```python
from build123d import *

# Parameters (mm, degrees)
F0_W      = 438.5
F0_H      = 130
F1_DEPTH  = 14
F2_W      = 30
F2_H      = 10
F3_DEPTH  = 130
F4_W      = 11
F4_H      = 16
F5_DEPTH  = 130
F6_W      = 42.5
F6_H      = 23.3528089888
F6_H_2    = 62.2471910113
F7_DEPTH  = 25
F8_R      = 2.5
F9_DEPTH  = 25
F10_R     = 2.5
F11_DEPTH = 468.501
F12_SIZE  = 3.49999


# Not quite as in the source:
# - a fillet or chamfer is up to 0.001 mm smaller than in the source, because OpenCascade refuses the exact size
# - a feature names something its author has since deleted; it is built from what else it names


with BuildPart() as f1:
    # F0 (on Front) → F1 (new body)
    with BuildSketch(Plane.XZ):
        with Locations((219.25, 65)):
            Rectangle(F0_W, F0_H)
    extrude(amount=F1_DEPTH)

    # F2 (on face) → F3 (join, through all)
    with BuildSketch(Plane.XY.offset(130)):
        with Locations((453.5, -9)):
            Rectangle(F2_W, F2_H)
        with Locations((-15, -9)):
            Rectangle(F2_W, F2_H)
    extrude(amount=-F3_DEPTH)

    # F4 (on face) → F5 (join, through all)
    with BuildSketch(Plane.XY.offset(130)):
        with Locations((5.5, 8)):
            Rectangle(F4_W, F4_H)
        with Locations((433, 8)):
            Rectangle(F4_W, F4_H)
    extrude(amount=-F5_DEPTH)

    # F6 (on face) → F7 (cut)
    with BuildSketch(Plane.XZ.offset(14)):
        Polygon((24.75, 120), (24.75, 95), (14.75, 95), (14.75, 57.7528089887), (24.75, 57.7528089887), (67.25, 57.7528089887), (67.25, 120), align=None)
        with Locations((46, 21.6764044942)):
            Rectangle(F6_W, F6_H)
        with Locations((101.4, 41.1235955055)):
            Rectangle(F6_W, F6_H_2)
        with Locations((143.9, 41.1235955055)):
            Rectangle(F6_W, F6_H_2)
        with Locations((101.4, 108.3235955056)):
            Rectangle(F6_W, F6_H)
        with Locations((143.9, 108.3235955056)):
            Rectangle(F6_W, F6_H)
        with Locations((199.3, 88.8764044943)):
            Rectangle(F6_W, F6_H_2)
        with Locations((241.8, 88.8764044943)):
            Rectangle(F6_W, F6_H_2)
        with Locations((199.3, 21.6764044942)):
            Rectangle(F6_W, F6_H)
        with Locations((241.8, 21.6764044942)):
            Rectangle(F6_W, F6_H)
        with Locations((297.2, 41.1235955055)):
            Rectangle(F6_W, F6_H_2)
        with Locations((339.7, 41.1235955055)):
            Rectangle(F6_W, F6_H_2)
        with Locations((339.7, 108.3235955056)):
            Rectangle(F6_W, F6_H)
        with Locations((297.2, 108.3235955056)):
            Rectangle(F6_W, F6_H)
        Polygon((416.35, 120), (373.85, 120), (373.85, 57.7528089887), (427.35, 57.7528089887), (427.35, 95), (416.35, 95), align=None)
        with Locations((395.1, 21.6764044942)):
            Rectangle(F6_W, F6_H)
    extrude(amount=-F7_DEPTH, mode=Mode.SUBTRACT)

    # F8 (on face) → F9 (cut)
    with BuildSketch(Plane(origin=(0, -4, 0), x_dir=(-1, 0, 0), z_dir=(0, 1, 0))):
        with Locations((-448.5, 115)):
            Circle(F8_R)
        with Locations((-448.5, 15)):
            Circle(F8_R)
        with Locations((10, 115)):
            Circle(F8_R)
        with Locations((10, 15)):
            Circle(F8_R)
    extrude(amount=-F9_DEPTH, mode=Mode.SUBTRACT)

    # F10 (on face) → F11 (cut, through all)
    with BuildSketch(Plane.YZ.offset(438.5)):
        with Locations((6, 115)):
            Circle(F10_R)
        with Locations((6, 15)):
            Circle(F10_R)
        with Locations((6, 65)):
            Circle(F10_R)
    extrude(amount=-F11_DEPTH, mode=Mode.SUBTRACT)

    # F12 (size 3.5 in the source; OpenCascade refuses exactly that, so slightly less here)
    f12_edges = [f1.edges().sort_by_distance(p)[0] for p in [
        (451, -14, 115),
        (451, -14, 15),
        (-7.5, -14, 115),
        (-7.5, -14, 15),
        (427.5, 3.5, 115),
        (427.5, 3.5, 65),
        (427.5, 3.5, 15),
        (11, 3.5, 115),
        (11, 3.5, 65),
        (11, 3.5, 15),
    ]]
    chamfer(f12_edges, length=F12_SIZE)


solid = f1.part
```
Geometry: final body of the model. Coordinates: model frame, mm. A direction names the side the tool comes from. Give positions to 0.01 mm unless a question says otherwise; leave off trailing zeros. Write each loop counter-clockwise with the first axis right and the second up, starting at its lowest first coordinate (ties: lowest second). Pieces come first, ordered by that corner, then holes.
1. Reachability of faces 4 (the conical face through (430.83, 5.421, 62.394)), 5 (the flat face through (416.35, -7, 107)), 6 (the flat face through (271, -5, 0)) from +Z, -Z, +X, -X, +Y, -Y: full face, straight path, thin tool, end or side. Return the list, or none.
2. Line query: probe 1 along X at (y, z) = (-3.5, 93); probe 2 along Z at (x, y) = (205, -6.25); probe 3 along X at (y, z) = (-3.25, 43). Output: solid intervals per line, ascending.
3. Section query A-A, the plane z = 83.5. Return loops of the section in (x, y), then the cut area to 3 significant figures.
4. Draft query along X for faces 1 (the flat face through (5, 16, 66)), 2 (the flat face through (20, -7, 95)), 3 (the flat face through (178.05, -7, 88)). Return one class per face: released by +X, released by -X, zero draft, split by the parting line, or undercut.
5. Section query B-B, the plane x = 102. Return loops of the section in (y, z), then the cut area to 3 significant figures.
6. Pin query (flat end, axial travel): P1, Ø24, axis at x = 452, z = 41, coming from the +Y side; P2, Ø1.5, axis at y = 10, z = 84.5, coming from the +X side; P3, Ø5, axis at y = 6, z = 84, coming from the -X side; P4, Ø5, axis at x = 213.5, y = 4.5, coming from the -Z side. Return the tip coordinate at first contact, or that it passes through.
7. Section query C-C, the plane z = 47. Return loops of the section in (x, y).
Computed:
1. face 4: none
1. face 5: +Y, -Y
1. face 6: -Z, +X, -X, +Y, -Y
2. probe 1: x = 0 to 14.75, 67.25 to 178.05, 263.05 to 373.85, 427.35 to 438.5
2. probe 2: z = 0 to 10, 33.35 to 57.75, 120 to 130
2. probe 3: x = 0 to 80.15, 165.15 to 275.95, 360.95 to 438.5
3. outline: (-30, -14) - (14.75, -14) - (14.75, 0) - (11, 0) - (11, 16) - (0, 16) - (0, -4) - (-30, -4) - close; (67.25, -14) - (178.05, -14) - (178.05, 0) - (67.25, 0) - close; (263.05, -14) - (373.85, -14) - (373.85, 0) - (263.05, 0) - close; (427.35, -14) - (468.5, -14) - (468.5, -4) - (438.5, -4) - (438.5, 16) - (427.5, 16) - (427.5, 0) - (427.35, 0) - close
3. area: 4,420 mm2
4. face 1: zero draft
4. face 2: undercut
4. face 3: undercut
5. outline: (-14, 0) - (0, 0) - (0, 10) - (-14, 10) - close; (-14, 72.25) - (0, 72.25) - (0, 96.65) - (-14, 96.65) - close; (-14, 120) - (0, 120) - (0, 130) - (-14, 130) - close
5. area: 622 mm2
6. P1: stops at y = -4
6. P2: stops at x = 438.5
6. P3: stops at x = 0
6. P4: passes through
7. outline: (-30, -14) - (80.15, -14) - (80.15, 0) - (11, 0) - (11, 16) - (0, 16) - (0, -4) - (-30, -4) - close; (165.15, -14) - (275.95, -14) - (275.95, 0) - (165.15, 0) - close; (360.95, -14) - (468.5, -14) - (468.5, -4) - (438.5, -4) - (438.5, 16) - (427.5, 16) - (427.5, 0) - (360.95, 0) - close
